Print and shaded views of the part. All mm, measured from the part's lowest x, y and z. Coordinates: 2 decimals unless noted, no trailing zeros. Loops run counter-clockwise (first coordinate to the right, second up) from the corner with the lowest first, then second, coordinate; pieces in that order, holes last. Notation, with made-up numbers: (-20.75, -22) -> (27.25, -22) arc R33 cw to (27.25, 14) -> close; hole circle Ø6 at (45.25, -13). An arc over 180 degrees is marked (long way). One line per question, with ' | ' between items. Start each with the question number.
1) Cut at C-C (z = 8). List the corners of the cut face in (x, y), plus the area to 3 significant figures.
2) Cut at A-A (z = 48.5). List the corners of the cut face in (x, y), plus the area to 3 significant figures.
3) Cut at B-B (x = 42). List the corners of the cut face in (y, z), plus the area to 3 significant figures.
4) Probe L1, parallel to X at y = 0.3, z = 47; L2, parallel to Z at x = 86, y = 2.25; L3, parallel to Z at x = 28, y = 2.35. List the from-to ranges inside material, lowest first. Write a range as from..to.
5) Cut at D-D (y = 0.8). Count the separate pieces of the cut face and the enclosed holes in it, plus the area to 3 significant figures.
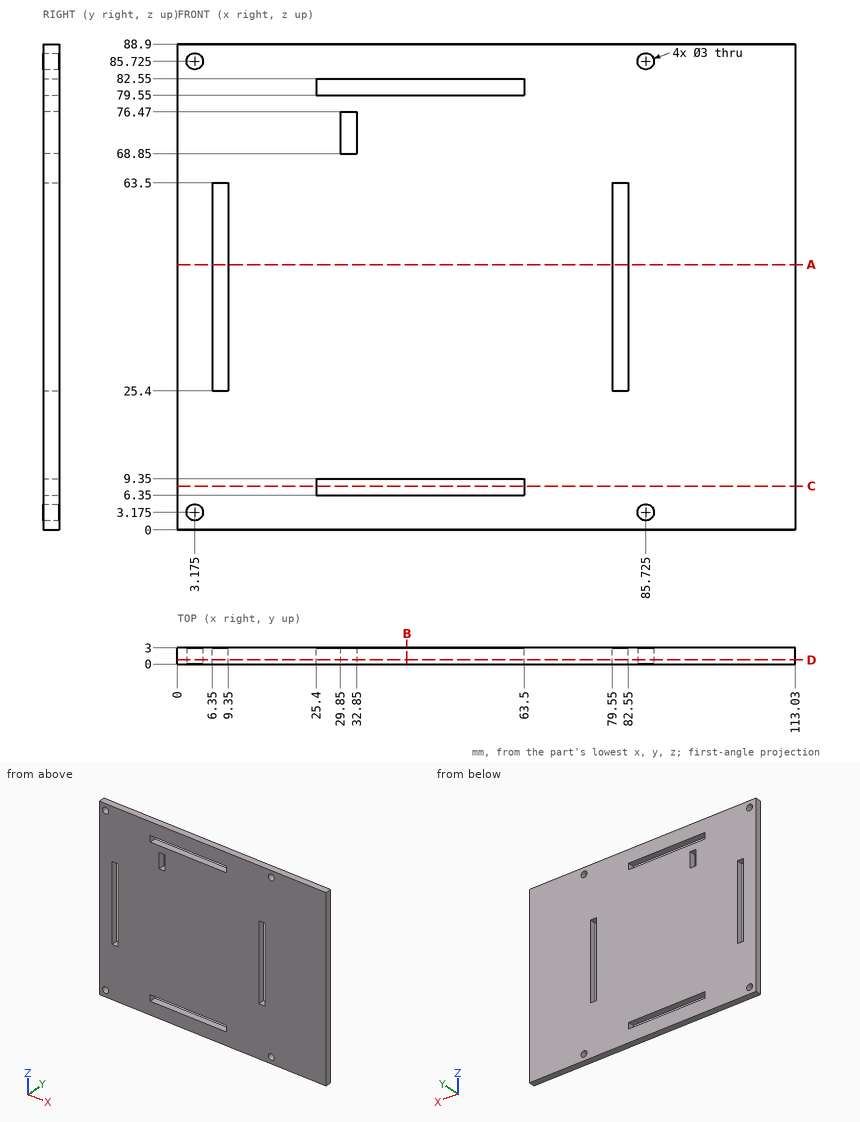
Reported:
1) outline: (0, 0) -> (25.4, 0) -> (25.4, 3) -> (0, 3) -> close; (63.5, 0) -> (113.03, 0) -> (113.03, 3) -> (63.5, 3) -> close | area: 225 mm²
2) outline: (0, 0) -> (6.35, 0) -> (6.35, 3) -> (0, 3) -> close; (9.35, 0) -> (79.55, 0) -> (79.55, 3) -> (9.35, 3) -> close; (82.55, 0) -> (113.03, 0) -> (113.03, 3) -> (82.55, 3) -> close | area: 321 mm²
3) outline: (0, 0) -> (3, 0) -> (3, 6.35) -> (0, 6.35) -> close; (0, 9.35) -> (3, 9.35) -> (3, 79.55) -> (0, 79.55) -> close; (0, 82.55) -> (3, 82.55) -> (3, 88.9) -> (0, 88.9) -> close | area: 249 mm²
4) L1: x = 0..6.35, 9.35..79.55, 82.55..113.03 | L2: z = 0..1.7, 4.65..84.25, 87.2..88.9 | L3: z = 0..6.35, 9.35..79.55, 82.55..88.9
5) separate pieces: 1 | enclosed holes: 9 | area: 9,540 mm²
